from build123d import *

# Parameters (mm, degrees)
SKETCH1_W           = 29.04
SKETCH1_H           = 23.1
SKETCH1_R           = 1
BOSS_EXTRUDE1_DEPTH = 2.5
SKETCH2_W           = 29.04
SKETCH2_H           = 2.5
BOSS_EXTRUDE2_DEPTH = 0.5
SKETCH3_W           = 29.04
SKETCH3_H           = 2.5
BOSS_EXTRUDE3_DEPTH = 0.5


with BuildPart() as part:
    # Sketch1 → Boss-Extrude1 (new body)
    with BuildSketch(Plane(origin=(0, 0, 0), x_dir=(1, 0, 0), z_dir=(0, 1, 0))):
        with Locations((-0.98, -0.45)):
            Rectangle(SKETCH1_W, SKETCH1_H)
        with Locations((-9.98, 8.55)):
            Circle(SKETCH1_R, mode=Mode.SUBTRACT)
        with Locations((8.02, 8.55)):
            Circle(SKETCH1_R, mode=Mode.SUBTRACT)
        with Locations((8.02, -9.45)):
            Circle(SKETCH1_R, mode=Mode.SUBTRACT)
        with Locations((-9.98, -9.45)):
            Circle(SKETCH1_R, mode=Mode.SUBTRACT)
    extrude(amount=BOSS_EXTRUDE1_DEPTH)

    # Sketch2 → Boss-Extrude2 (add)
    with BuildSketch(Plane(origin=(0, 0, -11.1), x_dir=(-1, 0, 0), z_dir=(0, 0, -1))):
        with Locations((0.98, 1.25)):
            Rectangle(SKETCH2_W, SKETCH2_H)
    extrude(amount=BOSS_EXTRUDE2_DEPTH)

    # Sketch3 → Boss-Extrude3 (add)
    with BuildSketch(Plane.XY.offset(12)):
        with Locations((-0.98, 1.25)):
            Rectangle(SKETCH3_W, SKETCH3_H)
    extrude(amount=BOSS_EXTRUDE3_DEPTH)


solid = part.part
For this review, take the finished solid that the model builds, in its own axes (mm). Give positions to 0.01 mm unless a question says otherwise; leave off trailing zeros. Write each loop counter-clockwise with the first axis right and the second up, starting at its lowest first coordinate (ties: lowest second). Pieces come first, ordered by that corner, then holes. Notation, with made-up numbers: (-2.5, 5.25) -> (36.5, 5.25) arc R24 cw to (36.5, 44.25) -> close; hole circle Ø11 at (6, 2.5). An arc over 180 degrees is marked (long way). Use CSV: the item, a comma, the result in double quotes.
Q1. Take a section at B-B, the plane y = 0.5. Write out the cut boundary in (x, z).
Conclusion:
outline,"(-15.5, -11.6) -> (13.54, -11.6) -> (13.54, 12.5) -> (-15.5, 12.5) -> close; hole circle Ø2 at (-9.98, -8.55); hole circle Ø2 at (-9.98, 9.45); hole circle Ø2 at (8.02, -8.55); hole circle Ø2 at (8.02, 9.45)"
Q2. Take a section at C-C, the plane x = -9.98. Write out the cut boundary in (y, z), then the cut area to 4 significant figures.
Conclusion:
outline,"(0, -11.6) -> (2.5, -11.6) -> (2.5, -9.55) -> (0, -9.55) -> close; (0, -7.55) -> (2.5, -7.55) -> (2.5, 8.45) -> (0, 8.45) -> close; (0, 10.45) -> (2.5, 10.45) -> (2.5, 12.5) -> (0, 12.5) -> close"
area,"50.25 mm2"
Q3. To check wall thickness, follow probe 1 along X at (y, z) = (1.85, 9.45); probe 2 along Z at (x, y) = (-9.98, 1.75); probe 3 along Z at (x, y) = (7.5, 1.65). State the ranges of each line that lie inside material, in increasing order. Write a range as [from, to].
Conclusion:
probe 1,"[-15.5, -10.98], [-8.98, 7.02], [9.02, 13.54]"
probe 2,"[-11.6, -9.55], [-7.55, 8.45], [10.45, 12.5]"
probe 3,"[-11.6, -9.4], [-7.7, 8.6], [10.3, 12.5]"
Q4. Take a section at A-A, the plane z = 9.45. Write out the cut boundary in (x, y).
Conclusion:
outline,"(-15.5, 0) -> (-10.98, 0) -> (-10.98, 2.5) -> (-15.5, 2.5) -> close; (-8.98, 0) -> (7.02, 0) -> (7.02, 2.5) -> (-8.98, 2.5) -> close; (9.02, 0) -> (13.54, 0) -> (13.54, 2.5) -> (9.02, 2.5) -> close"
Q5. Mouldability with a two-part tool opening along X and no side actions: class faces 1 (the face through (-1, 1, -11.6)), 2 (the face through (-15.5, 1, 0)), 3 (the face through (-10.77, 1.23, -7.94)) as pulls with the +X half, pulls with the -X half, needs draft (parallel to the pull), parting line crosses it, or undercut.
Conclusion:
face 1,"needs draft"
face 2,"pulls with the -X half"
face 3,"undercut"
Q6. For P1, Ø1.8, axis at x = -9.98, z = -8.55, coming from the -Y side, flat-tipped, find the tip position at first contact; note if it passes through.
Conclusion:
P1,"through"
